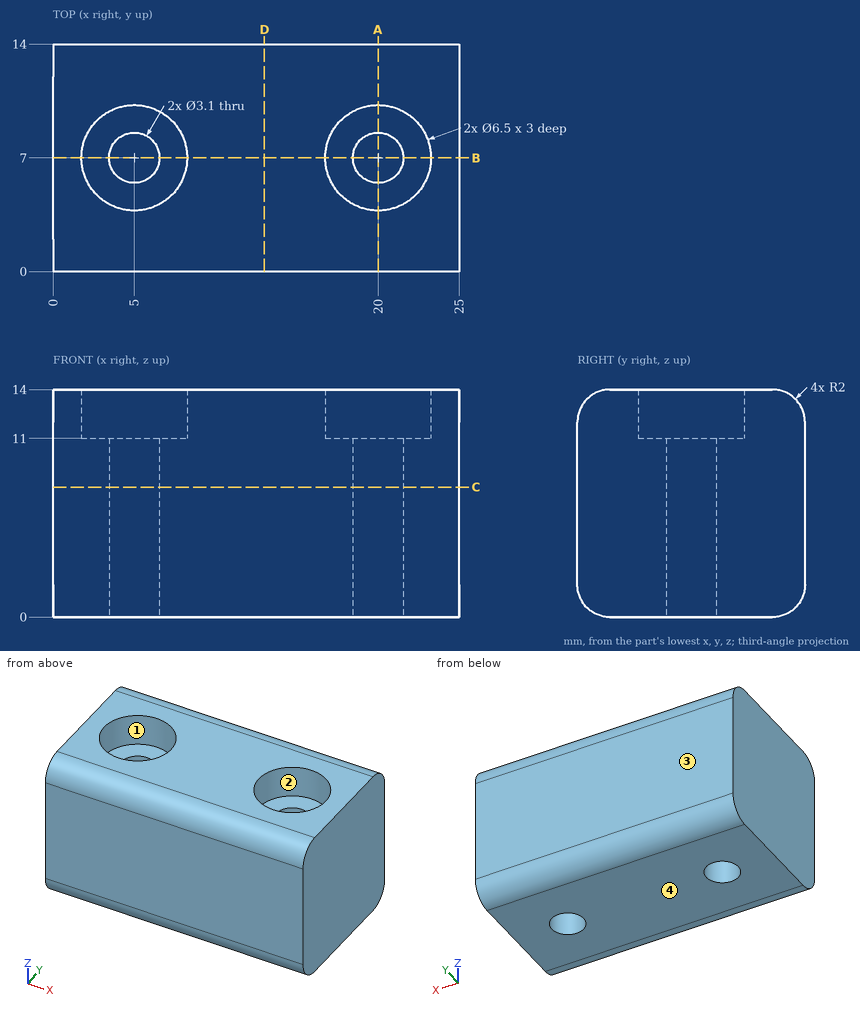
Print and shaded views of the part. All mm, measured from the part's lowest x, y and z. Give positions to 0.01 mm unless a question says otherwise; leave off trailing zeros. Loops run counter-clockwise (first coordinate to the right, second up) from the corner with the lowest first, then second, coordinate; pieces in that order, holes last.
1) Wall check: line 1 (X direction, y = 7, z = 10.25); line 2 (X direction, y = 7, z = 12.6); line 3 (Y direction, x = 5, z = 11.85). Give the ranges that are in metal, low to high.
2) Saw through at C-C (z = 8). Write the cut outline in (x, y), plus the area to 3 significant figures.
3) Saw through at D-D (x = 13). Write the cut outline in (y, z).
4) Pull direction Y, two halves, no side cores. Call the marked faces 1, 2, 3 and 4: +Y half, -Y half, draft (parallel to the pull), parting line (faces both ways), or undercut.
5) Saw through at A-A (x = 20). Write the cut outline in (y, z), plus the area to 3 significant figures.
6) Saw through at B-B (y = 7). Write the cut outline in (x, z), plus the area to 3 significant figures.
7) Flat gauge pin, fed straight in: pin 1 Ø2 at (x, y) = (20.5, 5.5) entering from +Z. Where does the tip first touch, or does it go through?
Answer block:
1. line 1: x = 0 to 3.45, 6.55 to 18.45, 21.55 to 25
1. line 2: x = 0 to 1.75, 8.25 to 16.75, 23.25 to 25
1. line 3: y = 0 to 3.75, 10.25 to 14
2. outline: (0, 0) - (25, 0) - (25, 14) - (0, 14) - close; hole circle Ø3.1 at (5, 7); hole circle Ø3.1 at (20, 7)
2. area: 335 mm2
3. outline: (0, 2) arc R2 ccw to (2, 0) - (12, 0) arc R2 ccw to (14, 2) - (14, 12) arc R2 ccw to (12, 14) - (2, 14) arc R2 ccw to (0, 12) - close
4. face 1: undercut
4. face 2: undercut
4. face 3: +Y half
4. face 4: draft
5. outline: (0, 2) arc R2 ccw to (2, 0) - (5.45, 0) - (5.45, 11) - (3.75, 11) - (3.75, 14) - (2, 14) arc R2 ccw to (0, 12) - close; (8.55, 0) - (12, 0) arc R2 ccw to (14, 2) - (14, 12) arc R2 ccw to (12, 14) - (10.25, 14) - (10.25, 11) - (8.55, 11) - close
5. area: 139 mm2
6. outline: (0, 0) - (3.45, 0) - (3.45, 11) - (1.75, 11) - (1.75, 14) - (0, 14) - close; (6.55, 0) - (18.45, 0) - (18.45, 11) - (16.75, 11) - (16.75, 14) - (8.25, 14) - (8.25, 11) - (6.55, 11) - close; (21.55, 0) - (25, 0) - (25, 14) - (23.25, 14) - (23.25, 11) - (21.55, 11) - close
6. area: 243 mm2
7. pin 1: stops at z = 11
